For this review, take the finished solid that the model builds, in its own axes (mm). A direction names the side the tool comes from. Give positions to 0.01 mm unless a question says otherwise; leave off trailing zeros. Write each loop counter-clockwise with the first axis right and the second up, starting at its lowest first coordinate (ties: lowest second). Pieces come first, ordered by that corner, then holes. Notation, with made-up numbers: M 8,-25 L 26,-25 A10 ccw 26,-6 Z; hole C 67,25 d8. An arc over 180 degrees is marked long. Write item = value, one per line.
```python
from build123d import *

# Parameters (mm, degrees)
SKETCH_1_W          = 12
SKETCH_1_H          = 33
EXTRUDE_1_DEPTH     = 10
SKETCH_3_OUTSIDE_W  = 21.302
SKETCH_3_OUTSIDE_H  = 19.302
CUT_EXTRUDE_1_DEPTH = 15.1
SKETCH_4_R          = 3
EXTRUDE_2_DEPTH     = 1.5
SKETCH_5_W          = 1
SKETCH_5_H          = 2
EXTRUDE_3_DEPTH     = 3
SKETCH_6_R          = 2
EXTRUDE_4_DEPTH     = 0.5
SKETCH_7_R          = 1.5
EXTRUDE_5_DEPTH     = 7.5
SKETCH_8_W          = 5.870249933
SKETCH_8_H          = 2.720447988
CUT_EXTRUDE_2_DEPTH = 7.5
FILLET_1_R          = 1
SKETCH_9_R          = 1
CUT_EXTRUDE_3_DEPTH = 23.721135535


with BuildPart() as part:
    # 草图1 → 凸台-拉伸1 (new body)
    with BuildSketch(Plane(origin=(0, 0, 0), x_dir=(1, 0, 0), z_dir=(0, 1, 0))):
        Rectangle(SKETCH_1_W, SKETCH_1_H)
    extrude(amount=EXTRUDE_1_DEPTH)

    # 草图3 outside → 切除-拉伸1 (cut)
    with BuildSketch(Plane.XY.offset(16.5)):
        with Locations((0, 5)):
            Rectangle(SKETCH_3_OUTSIDE_W, SKETCH_3_OUTSIDE_H)
        with BuildLine():
            Line((-3, 10), (3, 10))
            ThreePointArc((3, 10), (5.121320344, 9.121320344), (6, 7))
            Line((6, 7), (6, 3))
            ThreePointArc((6, 3), (5.121320344, 0.878679656), (3, 0))
            Line((3, 0), (-3, 0))
            ThreePointArc((-3, 0), (-5.121320344, 0.878679656), (-6, 3))
            Line((-6, 3), (-6, 7))
            ThreePointArc((-6, 7), (-5.121320344, 9.121320344), (-3, 10))
        make_face(mode=Mode.SUBTRACT)
    extrude(amount=-CUT_EXTRUDE_1_DEPTH, mode=Mode.SUBTRACT)

    # 草图4 → 凸台-拉伸2 (add)
    with BuildSketch(Plane.XY.offset(16.5)):
        with Locations((0, 5)):
            Circle(SKETCH_4_R)
    extrude(amount=EXTRUDE_2_DEPTH)

    # 草图5 → 凸台-拉伸3 (add)
    with BuildSketch(Plane.XY.offset(16.5)):
        with Locations((4.5, 5)):
            Rectangle(SKETCH_5_W, SKETCH_5_H)
        with Locations((-4.5, 5)):
            Rectangle(SKETCH_5_W, SKETCH_5_H)
    extrude(amount=EXTRUDE_3_DEPTH)

    # 草图6 → 凸台-拉伸4 (add)
    with BuildSketch(Plane(origin=(0, 10, 0), x_dir=(1, 0, 0), z_dir=(0, 1, 0))):
        with Locations(Location((0, 12.5, 0), (0, 0, 270))):
            Circle(SKETCH_6_R)
    extrude(amount=EXTRUDE_4_DEPTH)

    # 草图7 → 凸台-拉伸5 (add)
    with BuildSketch(Plane(origin=(0, 10.5, 0), x_dir=(1, 0, 0), z_dir=(0, 1, 0))):
        with Locations(Location((0, 12.5, 0), (0, 0, 270))):
            Circle(SKETCH_7_R)
    extrude(amount=EXTRUDE_5_DEPTH)

    # 草图8 → 切除-拉伸2 (cut)
    with BuildSketch(Plane(origin=(0, 18, 0), x_dir=(1, 0, 0), z_dir=(0, 1, 0))):
        with Locations((0.402921065, 10.139776006)):
            Rectangle(SKETCH_8_W, SKETCH_8_H)
    extrude(amount=-CUT_EXTRUDE_2_DEPTH, mode=Mode.SUBTRACT)

    # 圆角1
    fillet_1_edges = [part.edges().sort_by_distance(p)[0] for p in [
        (-6, 5, -16.5),
        (6, 5, -16.5),
    ]]
    fillet(fillet_1_edges, radius=FILLET_1_R)

    # 草图9 → 切除-拉伸3 (cut, through all)
    with BuildSketch(Plane(origin=(0, 10, 0), x_dir=(1, 0, 0), z_dir=(0, 1, 0))):
        with Locations(Location((-4.25, 14.75, 0), (0, 0, 270))):
            Circle(SKETCH_9_R)
        with Locations(Location((4.25, 14.75, 0), (0, 0, 270))):
            Circle(SKETCH_9_R)
    extrude(amount=-CUT_EXTRUDE_3_DEPTH, mode=Mode.SUBTRACT)


solid = part.part
```
1. We need section C-C, the plane z = 5.5. Write out the cut boundary in (x, y), then the cut area to 3 significant figures.
Responses:
outline = M -6,3 A3 ccw -3,0 L 3,0 A3 ccw 6,3 L 6,7 A3 ccw 3,10 L -3,10 A3 ccw -6,7 Z
area = 112 mm2
2. Insertion check: P1, Ø5, axis at x = -2, y = 16, coming from the +Z side; P2, Ø1.5, axis at x = -4, z = 4.5, coming from the -Y side; P3, Ø3.5, axis at x = -1, z = 8, coming from the +Y side. Each pin has a flat end and moves straight along its axis. Give the tip position at first contact, or say it passes through.
Responses:
P1 = -11.5
P2 = 0.01
P3 = 10
3. Machinability: for faces 1 (the face through (0, 5, 18)), 2 (the face through (-5.1, 0.86, 9.06)), 3 (the face through (-5.14, 9.1, 9.06)), 4 (the face through (0, 14, -11.5)), 5 (the face through (5.1, 9.14, 9.06)), which of the approach directions +Z, -Z, +X, -X, +Y, -Y give a long, thin tool a straight path to every point of the face, cutting with its end or side? Answer none if there is none.
Responses:
face_1 = +Z, +Y, -Y
face_2 = +Z, -X, -Y
face_3 = +Z, -X, +Y
face_4 = +Z, +X, -X, +Y
face_5 = +Z, +X, +Y
4. The part is to be moulded in two halves that separate along Z. For faces 6 (the face through (4.5, 6, 18)), 7 (the face through (-3.95, 5.07, -13.796)), 8 (the face through (-5.715, 5.07, -16.199)), say which applies: +Z half, -Z half, draft (parallel to the pull), parting line (faces both ways), or undercut.
Responses:
face_6 = draft
face_7 = undercut
face_8 = -Z half
5. For line 1 along X through (y, z) = (7, -14.75); line 2 along Y through (x, z) = (1, 4); line 3 along Z through (x, y) = (0, 8.5), list the stretches that pass through material, from the lowest coordinate up. Write a range as from..to.
Responses:
line_1 = -6..-5.25, -3.25..3.25, 5.25..6
line_2 = 0..10
line_3 = -16.5..16.5
6. We need section B-B, the plane y = 5. Write out the cut boundary in (x, z), then the cut area to 3 significant figures.
Responses:
outline = M -6,-15.5 A1 ccw -5,-16.5 L 5,-16.5 A1 ccw 6,-15.5 L 6,16.5 L 5,16.5 L 5,19.5 L 4,19.5 L 4,16.5 L 3,16.5 L 3,18 L -3,18 L -3,16.5 L -4,16.5 L -4,19.5 L -5,19.5 L -5,16.5 L -6,16.5 Z; hole C -4.25,-14.75 d2; hole C 4.25,-14.75 d2
area = 404 mm2
7. We need section D-D, the plane z = -12.5. Write out the cut boundary in (x, y).
Responses:
outline = M -6,0 L 6,0 L 6,10 L 2,10 L 2,10.5 L 1.5,10.5 L 1.5,18 L -1.5,18 L -1.5,10.5 L -2,10.5 L -2,10 L -6,10 Z
8. We need section A-A, the plane x = 0. Write out the cut boundary in (y, z).
Responses:
outline = M 0,-16.5 L 10,-16.5 L 10,-14.5 L 10.5,-14.5 L 10.5,-14 L 18,-14 L 18,-11.5 L 10.5,-11.5 L 10.5,-10.5 L 10,-10.5 L 10,16.5 L 8,16.5 L 8,18 L 2,18 L 2,16.5 L 0,16.5 Z
